Can you work these out from the model? Positions are in its coordinate system, mm. A direction names the side the tool comes from. Give positions to 0.01 mm unless a question says otherwise; leave off trailing zeros. Order: outer loops, then holes, each group sorted by start corner. A loop starts at its lowest first (then second) coordinate and runs counter-clockwise, first axis right, second up. Notation, with made-up numbers: (27, -30) -> (46, -30) arc R26 ccw to (46, 4) -> close; hole circle Ø3 at (-21.5, 55). An arc over 180 degrees is marked (long way). Answer as a JSON object with one key per item and string values.
```python
from build123d import *

# Parameters (mm, degrees)
F1_DEPTH = 50.8
F3_DEPTH = 25.4
F4_W     = 26.0413559154
F4_H     = 20.6534923054
F5_DEPTH = 7.62
F7_DEPTH = 25.4
F9_DEPTH = 25.4


with BuildPart() as f1:
    # F0 (on Front) → F1 (new body)
    with BuildSketch(Plane.XZ):
        Polygon((-42.4485914409, 0), (0, 0), (0, 62.4661669135), (-13.4870102629, 62.4661669135), (-13.4870102629, 13.6289829388), (-42.4485914409, 13.6289829388), align=None)
    extrude(amount=-F1_DEPTH)

    # F2 (on face) → F3 (cut)
    with BuildSketch(Plane.XY.offset(13.6289829388)):
        with BuildLine():
            ThreePointArc((-27.9678008519, 0), (-42.2028744607, 25.4), (-27.9678008519, 50.8))
            Line((-27.9678008519, 50.8), (-42.4485914409, 50.8))
            Line((-42.4485914409, 50.8), (-42.4485914409, 0))
            Line((-42.4485914409, 0), (-27.9678008519, 0))
        make_face()
    extrude(amount=-F3_DEPTH, mode=Mode.SUBTRACT)

    # F4 (on face) → F5 (cut)
    with BuildSketch(Plane.XZ):
        with Locations((-7.6980530284, 8.0353214871)):
            Rectangle(F4_W, F4_H)
    extrude(amount=-F5_DEPTH, mode=Mode.SUBTRACT)

    # F6 (on face) → F7 (cut)
    with BuildSketch(Plane.XY.offset(62.4661669135)):
        Polygon((0, 16.8692115694), (0, 25.4), (0, 35.7267484069), (-13.4870102629, 35.7267484069), (-13.4870102629, 16.8692115694), align=None)
    extrude(amount=-F7_DEPTH, mode=Mode.SUBTRACT)

    # F8 (on face) → F9 (cut)
    with BuildSketch(Plane(origin=(-13.4870102629, 0, 0), x_dir=(0, -1, 0), z_dir=(-1, 0, 0))):
        with BuildLine():
            Line((-16.8692115694, 37.0661669135), (-35.7267484069, 37.0661669135))
            ThreePointArc((-35.7267484069, 37.0661669135), (-26.2979799882, 27.6373984948), (-16.8692115694, 37.0661669135))
        make_face()
    extrude(amount=-F9_DEPTH, mode=Mode.SUBTRACT)


solid = f1.part
```
1. If we section it at C-C on z = 4: Please give me the cut outline in (x, y), then the cut area to 3 significant figures.
Worked answers:
{"outline": "(-27.97, 0) -> (-20.72, 0) -> (-20.72, 7.62) -> (0, 7.62) -> (0, 50.8) -> (-27.97, 50.8) arc R29.78 ccw to start", "area": "1,770 mm²"}
2. Please list where these lines run through material, in increasing order: L1, parallel to Y at x = -7.5, z = 45.5; L2, parallel to Z at x = -14.5, y = 25.5; L3, parallel to Z at x = -3, y = 26.
Worked answers:
{"L1": "0 to 16.87, 35.73 to 50.8", "L2": "0 to 13.63", "L3": "0 to 27.64"}
3. If we section it at B-B on y = 6.5: Please give me the cut outline in (x, z).
Worked answers:
{"outline": "(-35.44, 0) -> (-20.72, 0) -> (-20.72, 13.63) -> (-35.44, 13.63) -> close; (-13.49, 18.36) -> (0, 18.36) -> (0, 62.47) -> (-13.49, 62.47) -> close"}
4. For faces 1 (the face through (-7, 16.869, 50)), 2 (the face through (-20.719, 4, 7)), 3 (the face through (-11, 7.62, 9)), which set-ups out of +Z, -Z, +X, -X, +Y, -Y let a thin tool reach every point of the face, with its end or its side?
Worked answers:
{"face 1": "+Z, +X, -X", "face 2": "+Z, -Z, +X, -Y", "face 3": "-Z, +X, -Y"}
5. Will these pins go through, and if not, where does the flat tip stop? pin 1 Ø1.5 at (x, y) = (-20, 38) entering from +Z; pin 2 Ø4 at (y, z) = (4, 6) entering from +X; pin 3 Ø6 at (x, y) = (-5, 4) entering from -Z.
Worked answers:
{"pin 1": "z = 13.63", "pin 2": "x = -20.72", "pin 3": "z = 18.36"}
6. If we section it at A-A on z = 46.5: Please give me the cut outline in (x, y).
Worked answers:
{"outline": "(-13.49, 0) -> (0, 0) -> (0, 16.87) -> (-13.49, 16.87) -> close; (-13.49, 35.73) -> (0, 35.73) -> (0, 50.8) -> (-13.49, 50.8) -> close"}
7. If we mould it in two halves opening along Y, with no side actions, what happens to faces 4 (the face through (-13.487, 25, 27.5)), 5 (the face through (-6.84, 26.51, 27.64)), 6 (the face through (-24, 0, 7))? For each: +Y half, -Y half, draft (parallel to the pull), parting line (faces both ways), or undercut.
Worked answers:
{"face 4": "draft", "face 5": "undercut", "face 6": "-Y half"}
8. If we section it at D-D on x = -22.5: Please give me the cut outline in (y, z).
Worked answers:
{"outline": "(0, 0) -> (50.8, 0) -> (50.8, 13.63) -> (0, 13.63) -> close"}
